```python
from build123d import *

# Parameters (mm, degrees)
EXTRUDE_1_DEPTH = 4
SKETCH_3_R      = 2.5
EXTRUDE_2_DEPTH = 60
FILLET_2_R      = 0.12


with BuildPart() as part:
    # 草图1 → 凸台-拉伸1 (new body)
    with BuildSketch(Plane.XY):
        Polygon((0, 4.618802154), (-4, 2.309401077), (-4, -2.309401077), (0, -4.618802154), (4, -2.309401077), (4, 2.309401077), align=None)
    extrude(amount=EXTRUDE_1_DEPTH)

    # 草图2 → 切除-旋转1 (revolve, cut)
    with BuildSketch(Plane(origin=(0, 0, 0), x_dir=(0, 0, -1), z_dir=(1, 0, 0))):
        Polygon((0, 4.618802154), (0, 3.998802154), (-0.62, 4.618802154), align=None)
        Polygon((-3.38, 4.618802154), (-4, 3.998802154), (-4, 4.618802154), align=None)
    revolve(axis=Axis((0, 0, 0), (0, 0, -1)), mode=Mode.SUBTRACT)

    # 草图3 → 凸台-拉伸2 (add)
    with BuildSketch(Plane(origin=(0, 0, 0), x_dir=(-1, 0, 0), z_dir=(0, 0, -1))):
        Circle(SKETCH_3_R)
    extrude(amount=EXTRUDE_2_DEPTH)

    # 圆角2
    fillet_2_edges = [part.edges().sort_by_distance(p)[0] for p in [
        (2.5, 0, -60),
    ]]
    fillet(fillet_2_edges, radius=FILLET_2_R)


solid = part.part
```
Read the model definition and answer for the solid it produces. Units are mm, in the model's axes. A direction names the side the tool comes from. Round coordinates to 2 decimals unless told otherwise and drop trailing zeros. Write each loop counter-clockwise with the first axis right and the second up, starting at its lowest first coordinate (ties: lowest second). Pieces come first, ordered by that corner, then holes. Notation, with made-up numbers: (-28, 70) - (9, 70) arc R33 cw to (9, 103) - close; hole circle Ø8 at (11, -37.5). An arc over 180 degrees is marked (long way). Use CSV: the item, a comma, the result in double quotes.
Q1. Straight lines are drawn through the part: line 1 along Z through (x, y) = (-0.75, 3); line 2 along Y through (x, z) = (0, -35.5); line 3 along X through (y, z) = (-0.75, -35). For each, find the intervals that lie inside material, in ascending order.
Values:
line 1,"z = 0 to 4"
line 2,"y = -2.5 to 2.5"
line 3,"x = -2.38 to 2.38"
Q2. A tool of negligible diameter and unlimited length cuts with its end or side. For faces 1 (the flat face through (-4, 0, 2)), 2 (the cylindrical face through (0.54, -2.44, -29.52)), from which of +Z, -Z, +X, -X, +Y, -Y can it reach the whole face along a straight path? Write none if from no direction.
Values:
face 1,"+Z, -Z, -X, +Y, -Y"
face 2,"-Z"
Q3. Find section B-B, the plane z = -52.5. Write down the section's boundary in (x, y).
Values:
outline,"circle Ø5 at (0, 0)"
Q4. Each of these flat-tipped pins is pushed along its axis until it touches: pin 1 Ø1.5 at (x, y) = (-1, 3.5) entering from -Z; pin 2 Ø3 at (x, z) = (2, -5) entering from +Y; pin 3 Ø2 at (y, z) = (-1, -49) entering from -X. Where does it stop, or does it pass through?
Values:
pin 1,"stops at z = 0"
pin 2,"stops at y = 2.45"
pin 3,"stops at x = -2.5"
